The model under review builds one solid part; all positions refer to its coordinate system, in mm. A direction names the side the tool comes from. Coordinates: 2 decimals unless noted, no trailing zeros. Loops run counter-clockwise (first coordinate to the right, second up) from the corner with the lowest first, then second, coordinate; pieces in that order, holes last. Notation, with made-up numbers: (87.25, 49) - (146.25, 49) arc R36 ccw to (146.25, 83) - close; hole circle Ø1 at (1, 54). An arc over 180 degrees is marked (long way). Use a Markdown table: item, result. Add a question column.
1) The part is to be moulded in two halves that separate along X. For faces 1 (the cylindrical face through (44.49, 0.74, 149.47)), 2 (the flat face through (-4.756, 8, 67)), 3 (the flat face through (14, 6, 92.79)), 4 (the flat face through (4.8, 21, 68)), say which applies: pulls with the +X half, pulls with the -X half, needs draft (parallel to the pull), parting line crosses it, or undercut.
2) Add section A-A, the plane x = 0. Give the boundary of the cut face in (y, z).
3) Add section C-C, the plane z = 91.5. Give the boundary of the cut face in (x, y), and give its area (3 significant figures).
4) For faces 5 (the cylindrical face through (-38.72, 0.76, 140.73)), 6 (the flat face through (0, 12, 57.79)), 7 (the flat face through (0, 8, 58.35)), 8 (the flat face through (0, 12, 77.79)), list the 3-axis set-ups (+Z, -Z, +X, -X, +Y, -Y) from which the entire face can be reached by the end or side of a thin tool; tool diameter is ignored.
5) Clearance check with flat-ended pins moving along their axes: pin 1 (3.5 mm diameter, centred on x = 0, z = 63.3, fed in from +Y); pin 2 (7.5 mm diameter, centred on x = -1.5, z = 73, fed in from +Y); pin 3 (4.5 mm diameter, centred on x = 37.5, z = 67.32, fed in from +Y); pin 4 (10.5 mm diameter, centred on x = 4.5, y = 9.5, fed in from -Z). State where each tip first meets the part, or that it passes through.
6) Add section B-B, the plane y = 3.75. Give the boundary of the cut face in (x, z), and give its area (3 significant figures).
7) To check wall thickness, follow L1, parallel to X at y = 17, z = 81; L2, parallel to X at y = 10.5, z = 74; L3, parallel to Z at x = -1, y = 3.25. State the ranges of each line that lie inside material, in increasing order. Write a range as [from, to].
8) Add section D-D, the plane x = 22. Give the boundary of the cut face in (y, z), and give its area (4 significant figures).
```python
from build123d import *

# Parameters (mm, degrees)
EXTRUDE_1_DEPTH      = 1.5
SKETCH_2_W           = 32.36053695
SKETCH_2_H           = 20
EXTRUDE_2_DEPTH      = 18
SKETCH_3_W           = 3.3
SKETCH_3_H           = 0.56
SKETCH_3_W_2         = 0.5
SKETCH_3_W_3         = 1
EXTRUDE_4_DEPTH      = 3
SKETCH_6_W           = 4
SKETCH_6_H           = 15
EXTRUDE_7_DEPTH      = 20
CUT_EXTRUDE_START    = -4
CUT_EXTRUDE_3_DEPTH  = 4
CUT_EXTRUDE_4_DEPTH  = 4
SKETCH_12_R          = 1
CUT_EXTRUDE_9_DEPTH  = 71.381105419
SKETCH_14_R          = 1
CUT_EXTRUDE_10_DEPTH = 71.381105419
SKETCH_15_R          = 1
CUT_EXTRUDE_12_DEPTH = 71.381105419
SKETCH_16_W          = 9.556308291
SKETCH_16_H          = 18
CUT_EXTRUDE_13_DEPTH = 17
CUT_EXTRUDE_14_DEPTH = 161.738742996
SKETCH_18_R          = 2
CUT_EXTRUDE_15_DEPTH = 161.738742996


# Read off the part's stored shape, not the designer's step: 切除-拉伸3, 切除-拉伸4
with BuildPart() as part:
    # 草图1 → 凸台-拉伸1 (new body)
    with BuildSketch(Plane(origin=(0, 0, 104.816917971), x_dir=(1, 0, 0), z_dir=(0, 1, 0))):
        with BuildLine():
            Line((-37.5, -47.5), (37.5, -47.5))
            ThreePointArc((37.5, -47.5), (44.571067812, -44.571067812), (47.5, -37.5))
            Line((47.5, -37.5), (47.5, 37.5))
            ThreePointArc((47.5, 37.5), (44.571067812, 44.571067812), (37.5, 47.5))
            Line((37.5, 47.5), (-37.5, 47.5))
            ThreePointArc((-37.5, 47.5), (-44.571067812, 44.571067812), (-47.5, 37.5))
            Line((-47.5, 37.5), (-47.5, -37.5))
            ThreePointArc((-47.5, -37.5), (-44.571067812, -44.571067812), (-37.5, -47.5))
        make_face()
    extrude(amount=EXTRUDE_1_DEPTH)

    # 草图2 → 凸台-拉伸2 (add)
    with BuildSketch(Plane(origin=(0, 1.5, 104.816917971), x_dir=(1, 0, 0), z_dir=(0, 1, 0))):
        with Locations((0, 37.027280992)):
            Rectangle(SKETCH_2_W, SKETCH_2_H)
    extrude(amount=EXTRUDE_2_DEPTH)

    # 草图3 → 凸台-拉伸4 (add)
    with BuildSketch(Plane(origin=(0, 19.5, 62.644818489), x_dir=(1, 0, 0), z_dir=(0, 1, 0))):
        with Locations((2.15, 4.575181511)):
            Rectangle(SKETCH_3_W, SKETCH_3_H)
        with Locations((-2.15, 4.575181511)):
            Rectangle(SKETCH_3_W, SKETCH_3_H)
        with Locations((-0.25, 4.575181511)):
            Rectangle(SKETCH_3_W_2, SKETCH_3_H)
        with Locations((0.25, 4.575181511)):
            Rectangle(SKETCH_3_W_2, SKETCH_3_H)
        with Locations((4.3, 4.575181511)):
            Rectangle(SKETCH_3_W_3, SKETCH_3_H)
        with Locations((-4.3, 4.575181511)):
            Rectangle(SKETCH_3_W_3, SKETCH_3_H)
        Polygon((4.8, 4.295181511), (4.8, -15.144818489), (16.180268475, -15.144818489), (16.180268475, 4.855181511), (4.8, 4.855181511), align=None)
        Polygon((-4.8, -15.144818489), (-4.8, 4.295181511), (-4.8, 4.855181511), (-16.180268475, 4.855181511), (-16.180268475, -15.144818489), align=None)
    extrude(amount=EXTRUDE_4_DEPTH)

    # 草图6 → 凸台-拉伸7 (add)
    with BuildSketch(Plane(origin=(0, 1.5, 104.816917971), x_dir=(1, 0, 0), z_dir=(0, 1, 0))):
        with Locations((14.180268475, 19.527280992)):
            Rectangle(SKETCH_6_W, SKETCH_6_H)
        with Locations((-14.180268475, 19.527280992)):
            Rectangle(SKETCH_6_W, SKETCH_6_H)
    extrude(amount=EXTRUDE_7_DEPTH)

    # 切除-拉伸3 outline → 切除-拉伸3 (cut)
    with BuildSketch(Plane(origin=(16.180268475, 0, 62.644818489), x_dir=(0, 0, -1), z_dir=(1, 0, 0)).offset(CUT_EXTRUDE_START)):
        Polygon((-30.144818489, 21.5), (-30.144818489, 11.5), (-15.144818489, 21.5), align=None)
    extrude(amount=CUT_EXTRUDE_3_DEPTH, mode=Mode.SUBTRACT)

    # 切除-拉伸4 outline → 切除-拉伸4 (cut)
    with BuildSketch(Plane(origin=(-12.180268475, 0, 70.144818489), x_dir=(0, 0, -1), z_dir=(1, 0, 0)).offset(CUT_EXTRUDE_START)):
        Polygon((-22.644818489, 21.5), (-22.644818489, 11.5), (-7.644818489, 21.5), align=None)
    extrude(amount=CUT_EXTRUDE_4_DEPTH, mode=Mode.SUBTRACT)

    # 草图12 → 切除-拉伸9 (cut, through all)
    with BuildSketch(Plane(origin=(0, 1.5, 104.816917971), x_dir=(1, 0, 0), z_dir=(0, 1, 0))):
        with Locations(Location((-37.5, -37.5, 0), (0, 0, 270))):
            Circle(SKETCH_12_R)
        with Locations(Location((37.5, -37.5, 0), (0, 0, 270))):
            Circle(SKETCH_12_R)
        with Locations(Location((37.5, 37.5, 0), (0, 0, 270))):
            Circle(SKETCH_12_R)
    extrude(amount=-CUT_EXTRUDE_9_DEPTH, mode=Mode.SUBTRACT)

    # 草图14 → 切除-拉伸10 (cut, through all)
    with BuildSketch(Plane(origin=(0, 1.5, 104.816917971), x_dir=(1, 0, 0), z_dir=(0, 1, 0))):
        with Locations(Location((-37.5, 37.5, 0), (0, 0, 270))):
            Circle(SKETCH_14_R)
    extrude(amount=-CUT_EXTRUDE_10_DEPTH, mode=Mode.SUBTRACT)

    # 草图15 → 切除-拉伸12 (cut, through all)
    with BuildSketch(Plane(origin=(0, 1.5, 104.816917971), x_dir=(1, 0, 0), z_dir=(0, 1, 0))):
        with Locations(Location((-37.5, 2.027280992, 0), (0, 0, 270))):
            Circle(SKETCH_15_R)
        with Locations(Location((37.5, 2.027280992, 0), (0, 0, 270))):
            Circle(SKETCH_15_R)
    extrude(amount=-CUT_EXTRUDE_12_DEPTH, mode=Mode.SUBTRACT)

    # 草图16 → 切除-拉伸13 (cut)
    with BuildSketch(Plane(origin=(0, 0, 0), x_dir=(-1, 0, 0), z_dir=(0, -1, 0))):
        with Locations((-0.021845855, -67.349636979)):
            Rectangle(SKETCH_16_W, SKETCH_16_H)
    extrude(amount=-CUT_EXTRUDE_13_DEPTH, mode=Mode.SUBTRACT)

    # 草图17 → 切除-拉伸14 (cut, through all)
    with BuildSketch(Plane(origin=(0, 19.5, 0), x_dir=(1, 0, 0), z_dir=(0, 1, 0))):
        with BuildLine():
            ThreePointArc((0, -70.3523833), (-1, -71.3523833), (0, -72.3523833))
            Line((0, -72.3523833), (0, -71.3523833))
            Line((0, -71.3523833), (0, -70.3523833))
        make_face()
        with BuildLine():
            Line((0, -71.3523833), (0, -72.3523833))
            ThreePointArc((0, -72.3523833), (0.707106781, -72.059490081), (1, -71.3523833))
            ThreePointArc((1, -71.3523833), (0.707106781, -70.645276519), (0, -70.3523833))
            Line((0, -70.3523833), (0, -71.3523833))
        make_face()
        with BuildLine():
            ThreePointArc((0, -62.303923017), (-1, -63.303923017), (0, -64.303923017))
            Line((0, -64.303923017), (0, -63.303923017))
            Line((0, -63.303923017), (0, -62.303923017))
        make_face()
        with BuildLine():
            Line((0, -63.303923017), (0, -64.303923017))
            ThreePointArc((0, -64.303923017), (0.707106781, -64.011029798), (1, -63.303923017))
            ThreePointArc((1, -63.303923017), (0.707106781, -62.596816236), (0, -62.303923017))
            Line((0, -62.303923017), (0, -63.303923017))
        make_face()
    extrude(amount=-CUT_EXTRUDE_14_DEPTH, mode=Mode.SUBTRACT)

    # 草图18 → 切除-拉伸15 (cut, through all)
    with BuildSketch(Plane(origin=(0, 19.5, 0), x_dir=(1, 0, 0), z_dir=(0, 1, 0))):
        with Locations(Location((0, -63.303923017, 0), (0, 0, 270))):
            Circle(SKETCH_18_R)
        with Locations(Location((0, -71.3523833, 0), (0, 0, 270))):
            Circle(SKETCH_18_R)
        with Locations(Location((-37.5, -67.316917971, 0), (0, 0, 270))):
            Circle(SKETCH_18_R)
        with Locations(Location((37.5, -67.316917971, 0), (0, 0, 270))):
            Circle(SKETCH_18_R)
        with Locations(Location((37.5, -102.789636979, 0), (0, 0, 270))):
            Circle(SKETCH_18_R)
        with Locations(Location((-37.5, -102.789636979, 0), (0, 0, 270))):
            Circle(SKETCH_18_R)
        with Locations(Location((-37.5, -142.316917971, 0), (0, 0, 270))):
            Circle(SKETCH_18_R)
        with Locations(Location((37.5, -142.316917971, 0), (0, 0, 270))):
            Circle(SKETCH_18_R)
    extrude(amount=-CUT_EXTRUDE_15_DEPTH, mode=Mode.SUBTRACT)


solid = part.part
```
From the geometry:
| question | item | result |
|---|---|---|
| 1 | face 1 | pulls with the +X half |
| 1 | face 2 | undercut |
| 1 | face 3 | needs draft |
| 1 | face 4 | undercut |
| 2 | outline | (0, 57.32) - (1.5, 57.32) - (1.5, 57.79) - (22.5, 57.79) - (22.5, 58.35) - (19.5, 58.35) - (19.5, 61.3) - (17, 61.3) - (17, 58.35) - (0, 58.35) - close; (0, 76.35) - (17, 76.35) - (17, 73.35) - (19.5, 73.35) - (19.5, 77.79) - (1.5, 77.79) - (1.5, 152.32) - (0, 152.32) - close; (17, 65.3) - (19.5, 65.3) - (19.5, 69.35) - (17, 69.35) - close |
| 3 | outline | (-47.5, 0) - (47.5, 0) - (47.5, 1.5) - (16.18, 1.5) - (16.18, 12.36) - (12.18, 12.36) - (12.18, 1.5) - (-12.18, 1.5) - (-12.18, 12.36) - (-16.18, 12.36) - (-16.18, 1.5) - (-47.5, 1.5) - close |
| 3 | area | 229 mm^2 |
| 4 | face 5 | +Y, -Y |
| 4 | face 6 | -Z, +X, -X, +Y |
| 4 | face 7 | -Y |
| 4 | face 8 | +Z, +Y |
| 5 | pin 1 | passes through |
| 5 | pin 2 | stops at y = 22.5 |
| 5 | pin 3 | stops at y = 1.5 |
| 5 | pin 4 | stops at z = 57.79 |
| 6 | outline | (-16.18, 57.79) - (16.18, 57.79) - (16.18, 92.79) - (12.18, 92.79) - (12.18, 77.79) - (-12.18, 77.79) - (-12.18, 92.79) - (-16.18, 92.79) - close; hole (-4.76, 58.35) - (4.8, 58.35) - (4.8, 76.35) - (-4.76, 76.35) - close |
| 6 | area | 595 mm^2 |
| 7 | L1 | x = [-16.18, -12.18], [12.18, 16.18] |
| 7 | L2 | x = [-16.18, -4.76], [4.8, 16.18] |
| 7 | L3 | z = [57.79, 58.35], [76.35, 77.79] |
| 8 | outline | (0, 57.32) - (1.5, 57.32) - (1.5, 152.32) - (0, 152.32) - close |
| 8 | area | 142.5 mm^2 |
